Answer from the drawing. Dimensions are ordinates in mm from the lowest x, y and z of the part. Coordinates: 2 decimals unless noted, no trailing zeros. Write each loop counter-clockwise with the first axis right and the second up, starting at its lowest first coordinate (ties: lowest second). Pieces come first, ordered by that corner, then holes. Notation, with made-up numbers: (-38.5, 74) - (-16.5, 74) arc R13 cw to (-16.5, 86) - close; hole circle Ø10 at (-35.75, 18). An arc over 180 degrees is marked (long way). Answer as a JSON object with one key per item and string values. Group by question number.
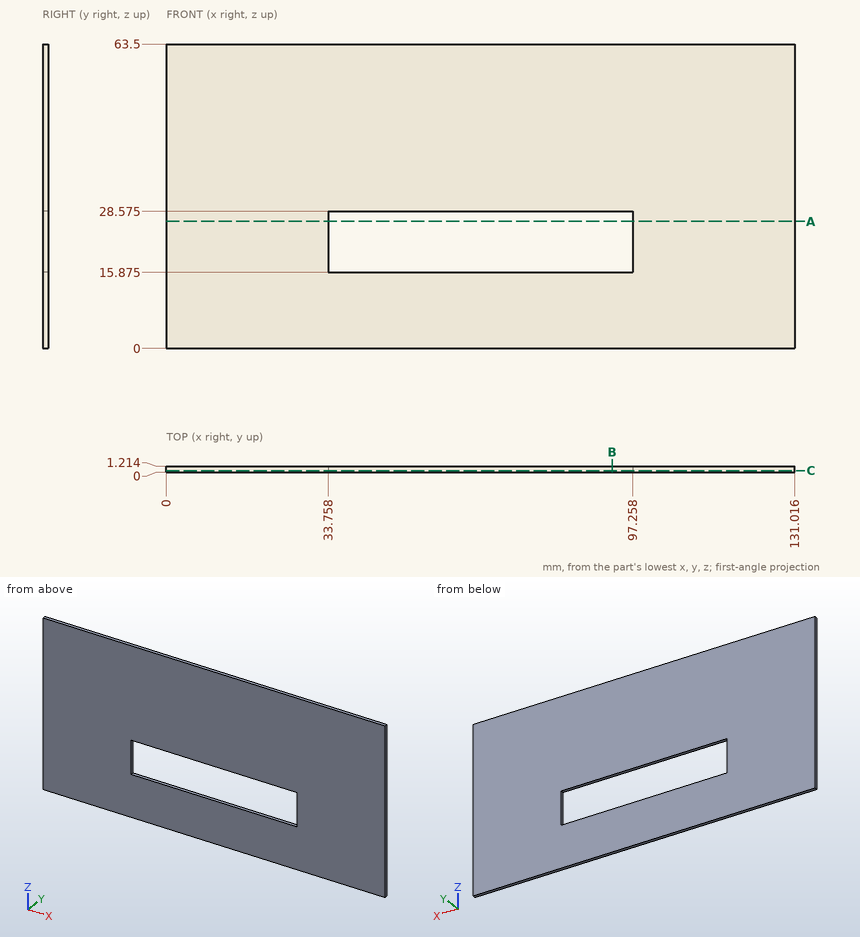
Q1. Section A-A on z = 26.5 is taken. Determine the outline of the cut face in (x, y).
Q2. Section C-C on y = 0.35 is taken. Determine the outline of the cut face in (x, z) (1 decimal).
Q3. Section B-B on x = 93 is taken. Determine the outline of the cut face in (y, z) (1 decimal).
Q4. Consider L1, parallel to X at y = 0.3, z = 21.5; L2, parallel to Z at x = 64, y = 1.1 (1 decimal). Determine where each line is inside the solid, lowest interval first. Write a range as from..to.
Numbers:
{
 "1": {"outline": "(0, 0) - (33.76, 0) - (33.76, 1.21) - (0, 1.21) - close; (97.26, 0) - (131.02, 0) - (131.02, 1.21) - (97.26, 1.21) - close"},
 "2": {"outline": "(0, 0) - (131, 0) - (131, 63.5) - (0, 63.5) - close; hole (33.8, 15.9) - (97.3, 15.9) - (97.3, 28.6) - (33.8, 28.6) - close"},
 "3": {"outline": "(0, 0) - (1.2, 0) - (1.2, 15.9) - (0, 15.9) - close; (0, 28.6) - (1.2, 28.6) - (1.2, 63.5) - (0, 63.5) - close"},
 "4": {"L1": "x = 0..33.76, 97.26..131.02", "L2": "z = 0..15.9, 28.6..63.5"}
}
